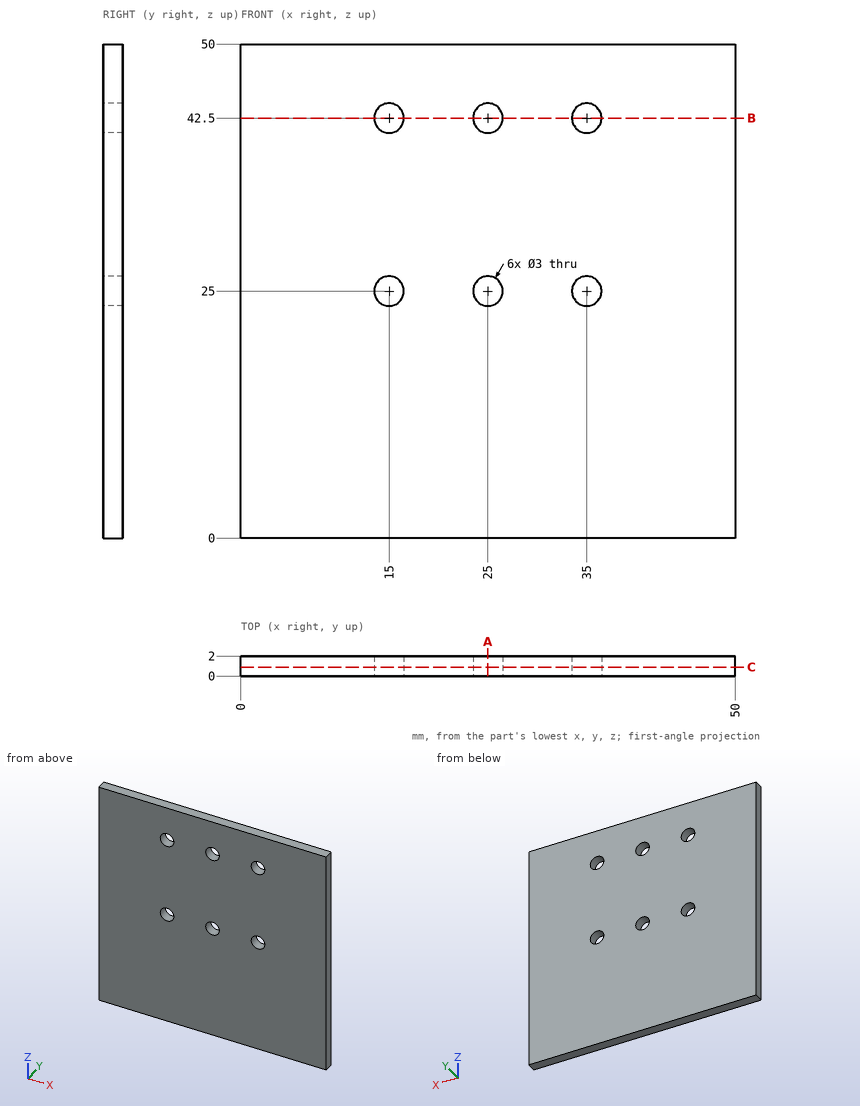
Design review of the part shown in the three views and the two pictorial views. Dimensions are in mm from the part's minimum x, y and z. Give positions to 0.01 mm unless a question says otherwise; leave off trailing zeros. Loops run counter-clockwise (first coordinate to the right, second up) from the corner with the lowest first, then second, coordinate; pieces in that order, holes last. Notation, with made-up numbers: M 49,37 L 75,37 A27 cw 75,56 Z; hole C 15,52 d5. An arc over 180 degrees is marked long. Put each result on its own line as item: value. Start each with the question number.
(1) Wall thickness on L1, parallel to Z at x = 35, y = 1.1; L2, parallel to X at y = 0.6, z = 42.5: over which ranges is each line inside the solid? List them lowest first.
(2) Add section C-C, the plane y = 0.9. Write out the cut boundary in (x, z), then the cut area to 3 significant figures.
(3) Add section A-A, the plane x = 25. Write out the cut boundary in (y, z), then the cut area to 3 significant figures.
(4) Add section B-B, the plane z = 42.5. Write out the cut boundary in (x, y).
Result:
1. L1: z = 0 to 23.5, 26.5 to 41, 44 to 50
1. L2: x = 0 to 13.5, 16.5 to 23.5, 26.5 to 33.5, 36.5 to 50
2. outline: M 0,0 L 50,0 L 50,50 L 0,50 Z; hole C 15,25 d3; hole C 15,42.5 d3; hole C 25,25 d3; hole C 25,42.5 d3; hole C 35,25 d3; hole C 35,42.5 d3
2. area: 2,460 mm^2
3. outline: M 0,0 L 2,0 L 2,23.5 L 0,23.5 Z; M 0,26.5 L 2,26.5 L 2,41 L 0,41 Z; M 0,44 L 2,44 L 2,50 L 0,50 Z
3. area: 88.0 mm^2
4. outline: M 0,0 L 13.5,0 L 13.5,2 L 0,2 Z; M 16.5,0 L 23.5,0 L 23.5,2 L 16.5,2 Z; M 26.5,0 L 33.5,0 L 33.5,2 L 26.5,2 Z; M 36.5,0 L 50,0 L 50,2 L 36.5,2 Z
